```python
from build123d import *

# Parameters (mm, degrees)
BOSS_EXTRUDE1_DEPTH = 3
SKETCH2_R           = 1
SKETCH2_W           = 6
SKETCH2_H           = 12
CUT_EXTRUDE1_DEPTH  = 3


with BuildPart() as part:
    # Sketch1 → Boss-Extrude1 (new body)
    with BuildSketch(Plane(origin=(0, 0, 0), x_dir=(1, 0, 0), z_dir=(0, 1, 0))):
        Polygon((-41, -41), (-17.5, -41), (-17.5, -38), (17.5, -38), (17.5, -41), (41, -41), (41, -17.5), (38, -17.5), (38, 17.5), (41, 17.5), (41, 41), (17.5, 41), (17.5, 38), (-17.5, 38), (-17.5, 41), (-41, 41), (-41, 17.5), (-38, 17.5), (-38, -17.5), (-41, -17.5), align=None)
    extrude(amount=BOSS_EXTRUDE1_DEPTH)

    # Sketch2 → Cut-Extrude1 (cut)
    with BuildSketch(Plane(origin=(0, 3, 0), x_dir=(1, 0, 0), z_dir=(0, 1, 0))):
        with Locations((0, 7.5)):
            Circle(SKETCH2_R)
        with Locations((0, -7.5)):
            Circle(SKETCH2_R)
        Rectangle(SKETCH2_W, SKETCH2_H)
    extrude(amount=-CUT_EXTRUDE1_DEPTH, mode=Mode.SUBTRACT)


solid = part.part
```
Read the model definition and answer for the solid it produces. Units are mm, in the model's axes. A direction names the side the tool comes from. Coordinates: 2 decimals unless noted, no trailing zeros. Write each loop counter-clockwise with the first axis right and the second up, starting at its lowest first coordinate (ties: lowest second). Pieces come first, ordered by that corner, then holes. Notation, with made-up numbers: (70, -29.75) -> (100, -29.75) arc R13 cw to (100, -14.75) -> close; hole circle Ø7 at (-8, 39). An arc over 180 degrees is marked (long way). Return JSON: item names as keys, results as strings.
1. Find the intervals of material crossed by line 1 along Z through (x, y) = (0, 1.4); line 2 along X through (y, z) = (1.1, 7.5); line 3 along Z through (x, y) = (-9.5, 0.95), in increasing order. Write a range as from..to.
Found:
{"line 1": "-38..-8.5, -6.5..-6, 6..6.5, 8.5..38", "line 2": "-38..-1, 1..38", "line 3": "-38..38"}
2. Determine the mould class of faces 4 (the face through (-17.5, 1, 40)), 5 (the face through (-1, 0, -10)), 6 (the face through (-41, 1, 29)) for opening direction X: pulls with the +X half, pulls with the -X half, needs draft (parallel to the pull), parting line crosses it, or undercut.
Found:
{"face 4": "undercut", "face 5": "needs draft", "face 6": "pulls with the -X half"}
3. A cutting plane is placed at D-D (z = -4.5). Determine the outline of the cut face in (x, y), and give its area (3 significant figures).
Found:
{"outline": "(-38, 0) -> (-3, 0) -> (-3, 3) -> (-38, 3) -> close; (3, 0) -> (38, 0) -> (38, 3) -> (3, 3) -> close", "area": "210 mm2"}
4. A tool of negligible diameter and unlimited length cuts with its end or side. For faces 1 (the face through (38, 1, 0)), 2 (the face through (-3, 2, 0)), 3 (the face through (0, 1, -38)), from which of +Z, -Z, +X, -X, +Y, -Y can it reach the whole face along a straight path? Write none if from no direction.
Found:
{"face 1": "+X, +Y, -Y", "face 2": "+Y, -Y", "face 3": "-Z, +Y, -Y"}
5. A cutting plane is placed at A-A (z = 7.5). Determine the outline of the cut face in (x, y).
Found:
{"outline": "(-38, 0) -> (-1, 0) -> (-1, 3) -> (-38, 3) -> close; (1, 0) -> (38, 0) -> (38, 3) -> (1, 3) -> close"}
6. A cutting plane is placed at B-B (x = 0). Determine the outline of the cut face in (y, z), and give its area (3 significant figures).
Found:
{"outline": "(0, -38) -> (3, -38) -> (3, -8.5) -> (0, -8.5) -> close; (0, -6.5) -> (3, -6.5) -> (3, -6) -> (0, -6) -> close; (0, 6) -> (3, 6) -> (3, 6.5) -> (0, 6.5) -> close; (0, 8.5) -> (3, 8.5) -> (3, 38) -> (0, 38) -> close", "area": "180 mm2"}
7. A cutting plane is placed at C-C (y = 0.9). Determine the outline of the cut face in (x, z).
Found:
{"outline": "(-41, -41) -> (-17.5, -41) -> (-17.5, -38) -> (17.5, -38) -> (17.5, -41) -> (41, -41) -> (41, -17.5) -> (38, -17.5) -> (38, 17.5) -> (41, 17.5) -> (41, 41) -> (17.5, 41) -> (17.5, 38) -> (-17.5, 38) -> (-17.5, 41) -> (-41, 41) -> (-41, 17.5) -> (-38, 17.5) -> (-38, -17.5) -> (-41, -17.5) -> close; hole (-3, -6) -> (3, -6) -> (3, 6) -> (-3, 6) -> close; hole circle Ø2 at (0, -7.5); hole circle Ø2 at (0, 7.5)"}
8. Each of these flat-tipped pins is pushed along its axis until it touches: P1, Ø2.5, axis at x = 0, z = 7.5, coming from the -Y side; P2, Ø1.5, axis at x = -0.5, y = 2, coming from the -Z side; P3, Ø0.9, axis at y = 2, z = 6.5, coming from the +X side. Where does it stop, or does it pass through?
Found:
{"P1": "y = 0", "P2": "z = -38", "P3": "x = 38"}
